```python
from build123d import *

# Parameters (mm, degrees)
SKETCH1_W               = 600
SKETCH1_H               = 100
BOSS_EXTRUDE1_DEPTH     = 50
SKETCH2_W               = 30
SKETCH2_H               = 100
CUT_EXTRUDE1_DEPTH      = 100
CUT_EXTRUDE3_DEPTH      = 610.590026165
CUT_EXTRUDE3_DEPTH_BACK = 610.590026165
SKETCH3_R               = 10


with BuildPart() as part:
    # Sketch1 → Boss-Extrude1 (new body)
    with BuildSketch(Plane.XY):
        with Locations((300, 50)):
            Rectangle(SKETCH1_W, SKETCH1_H)
    extrude(amount=BOSS_EXTRUDE1_DEPTH)

    # Sketch2 → Cut-Extrude1 (cut)
    with BuildSketch(Plane(origin=(600, 0, 0), x_dir=(0, 0, -1), z_dir=(1, 0, 0))):
        with Locations((-25, 50)):
            Rectangle(SKETCH2_W, SKETCH2_H)
    extrude(amount=-CUT_EXTRUDE1_DEPTH, mode=Mode.SUBTRACT)

    # Sketch3 → Cut-Extrude3 (cut, two sides: drawn at the far end of the back side and taken through both)
    with BuildSketch(Plane.XY.offset(10).offset(-CUT_EXTRUDE3_DEPTH_BACK)):
        with Locations((550, 51.950023211)):
            Circle(SKETCH3_R)
    extrude(amount=CUT_EXTRUDE3_DEPTH + CUT_EXTRUDE3_DEPTH_BACK, mode=Mode.SUBTRACT)


solid = part.part
```
For this review, take the finished solid that the model builds, in its own axes (mm). A direction names the side the tool comes from. Coordinates: 2 decimals unless noted, no trailing zeros. Write each loop counter-clockwise with the first axis right and the second up, starting at its lowest first coordinate (ties: lowest second). Pieces come first, ordered by that corner, then holes. Notation, with made-up numbers: (88, 27) - (145, 27) arc R24 cw to (145, 56) - close; hole circle Ø9 at (48, -7). An arc over 180 degrees is marked (long way). Answer in a Markdown table with one row per item. Add a question column.
Q1. We need section A-A, the plane x = 550. State the section outline as (y, z) points.
Q2. For P1, Ø3, axis at y = 63, z = 13.5, coming from the +X side, flat-tipped, find the tip position at first contact; note if it passes through.
Q3. We need section C-C, the plane z = 18.5. State the section outline as (x, y) points.
Q4. We need section B-B, the plane y = 89.5. State the section outline as (x, z) points, and give its area (3 significant figures).
Q5. Draft analysis for pull direction X (two halves, no side actions). For faces 1 (the cylindrical face through (559.54, 54.95, 4.93)), 2 (the flat face through (0, 49, 25)), 3 (the flat face through (296, 51, 0)), 4 (the flat face through (600, 49, 5)), state which applies: +X half, -X half, draft (parallel to the pull), parting line (faces both ways), or undercut.
Q6. For probe 1 along Y at (x, z) = (550, 7); probe 2 along X at (y, z) = (19, 31); probe 3 along X at (y, z) = (48.5, 3.5), list the stretches that pass through material, from the lowest coordinate up.
Q7. Tool access review of faces 5 (the flat face through (551, 38, 40)), 6 (the cylindrical face through (559.54, 54.95, 44.93)): name each direction out of +Z, -Z, +X, -X, +Y, -Y from which nothing blocks a thin tool from reaching the whole face with its end or side.
Answer list:
| question | item | result |
|---|---|---|
| 1 | outline | (0, 0) - (41.95, 0) - (41.95, 10) - (0, 10) - close; (0, 40) - (41.95, 40) - (41.95, 50) - (0, 50) - close; (61.95, 0) - (100, 0) - (100, 10) - (61.95, 10) - close; (61.95, 40) - (100, 40) - (100, 50) - (61.95, 50) - close |
| 2 | P1 | stops at x = 500 |
| 3 | outline | (0, 0) - (500, 0) - (500, 100) - (0, 100) - close |
| 4 | outline | (0, 0) - (600, 0) - (600, 10) - (500, 10) - (500, 40) - (600, 40) - (600, 50) - (0, 50) - close |
| 4 | area | 27,000 mm2 |
| 5 | face 1 | undercut |
| 5 | face 2 | -X half |
| 5 | face 3 | draft |
| 5 | face 4 | +X half |
| 6 | probe 1 | y = 0 to 41.95, 61.95 to 100 |
| 6 | probe 2 | x = 0 to 500 |
| 6 | probe 3 | x = 0 to 540.61, 559.39 to 600 |
| 7 | face 5 | +X, +Y, -Y |
| 7 | face 6 | +Z, -Z |
